from build123d import *

# Parameters (mm, degrees)
SKETCH1_R                = 12.5
BOSS_EXTRUDE1_DEPTH      = 150
BOSS_EXTRUDE2_START      = 75
SKETCH2_W                = 40
SKETCH2_H                = 30
BOSS_EXTRUDE2_DEPTH      = 5
BOSS_EXTRUDE2_DEPTH_BACK = 5


with BuildPart() as part:
    # Sketch1 → Boss-Extrude1 (new body)
    with BuildSketch(Plane.XY):
        Circle(SKETCH1_R)
    extrude(amount=BOSS_EXTRUDE1_DEPTH)

    # Sketch2 → Boss-Extrude2 (add, two sides)
    with BuildSketch(Plane.XY.offset(BOSS_EXTRUDE2_START)) as boss_extrude2_sk:
        Rectangle(SKETCH2_W, SKETCH2_H)
    extrude(amount=BOSS_EXTRUDE2_DEPTH)
    extrude(boss_extrude2_sk.sketch, amount=-BOSS_EXTRUDE2_DEPTH_BACK)


solid = part.part
Verification items for the finished model (mm, model axes). A direction names the side the tool comes from. Give positions to 0.01 mm unless a question says otherwise; leave off trailing zeros. Loops run counter-clockwise (first coordinate to the right, second up) from the corner with the lowest first, then second, coordinate; pieces in that order, holes last.
1. Cross-section at C-C on z = 87. Record the cut outline in (x, y).
Derived:
outline: circle Ø25 at (0, 0)
2. Cross-section at B-B on x = 0. Record the cut outline in (y, z).
Derived:
outline: (-15, 70) - (-12.5, 70) - (-12.5, 0) - (12.5, 0) - (12.5, 70) - (15, 70) - (15, 80) - (12.5, 80) - (12.5, 150) - (-12.5, 150) - (-12.5, 80) - (-15, 80) - close
3. Release check for a two-part mould opening along X. For faces 3 (the flat face through (-14, 0, 80)), 4 (the flat face through (20, 0, 75)), 5 (the cylindrical face through (11.923, 3.755, 114.51)) record: +X half, -X half, draft (parallel to the pull), parting line (faces both ways), or undercut.
Derived:
face 3: draft
face 4: +X half
face 5: parting line
4. Material ranges on probe 1 along Z at (x, y) = (-7, 11.25); probe 2 along X at (y, z) = (-0.5, 37.5); probe 3 along X at (y, z) = (-8, 28.5), recorded low to high.
Derived:
probe 1: z = 70 to 80
probe 2: x = -12.49 to 12.49
probe 3: x = -9.6 to 9.6
5. Tool access check on faces 1 (the flat face through (0, 0, 0)), 2 (the cylindrical face through (11.923, 3.755, 34.51)). Record the directions out of +Z, -Z, +X, -X, +Y, -Y that give a thin tool (end or side, any length) a straight path to the whole face; none if there is none.
Derived:
face 1: -Z, +X, -X, +Y, -Y
face 2: -Z
6. Cross-section at D-D on x = 16. Record the cut outline in (y, z), and give its area (3 significant figures).
Derived:
outline: (-15, 70) - (15, 70) - (15, 80) - (-15, 80) - close
area: 300 mm2
7. Go/stop test with flat-tipped pins: P1, Ø1.5, axis at x = -9, z = 91, coming from the +Y side; P2, Ø10, axis at y = 10.5, z = 60.5, coming from the +X side (3 decimals); P3, Ø8, axis at x = 3.5, z = 88, coming from the -Y side; P4, Ø12, axis at y = 6, z = 82.5, coming from the -X side. Record where each tip stops, or that it passes through.
Derived:
P1: stops at y = 9.39
P2: stops at x = 11.225
P3: stops at y = -12.5
P4: stops at x = -20
8. Cross-section at A-A on y = 0. Record the cut outline in (x, z), and give its area (3 significant figures).
Derived:
outline: (-20, 70) - (-12.5, 70) - (-12.5, 0) - (12.5, 0) - (12.5, 70) - (20, 70) - (20, 80) - (12.5, 80) - (12.5, 150) - (-12.5, 150) - (-12.5, 80) - (-20, 80) - close
area: 3,900 mm2
